For this review, take the finished solid that the model builds, in its own axes (mm). Coordinates: 2 decimals unless noted, no trailing zeros. Write each loop counter-clockwise with the first axis right and the second up, starting at its lowest first coordinate (ties: lowest second). Pieces come first, ordered by that corner, then holes. Notation, with made-up numbers: (49.5, 75.25) -> (81.5, 75.25) arc R7 ccw to (81.5, 82.25) -> close; hole circle Ø7 at (14, 58). An arc over 180 degrees is marked (long way). Put each result on its own line as item: value. Start each with the question number.
Item 1: Consider section C-C on x = 840. Give the boundary of the cut face in (y, z) (3 decimals), and give its area (3 significant figures).
Item 2: To check wall thickness, follow L1, parallel to X at y = 44.45, z = 6; L2, parallel to Y at x = 1365.25, z = 8; L3, parallel to X at y = 758.5, z = 14.75. State the ranges of each line that lie inside material, in increasing order.
Item 3: Consider section A-A on y = 698.5. Give the boundary of the cut face in (x, z) (3 decimals), and give its area (3 significant figures).
Item 4: Consider section B-B on z = 3.25. Give the boundary of the cut face in (x, y) (3 decimals).
Item 5: Insertion check: P1, Ø10, axis at x = 1365.25, y = 44.45, coming from the -Z side. The pin has a flat end and moves straight along its axis. Give the tip position at first contact, or say it passes through.
Autodesk Inventor part; units mm, degrees
ref_plane "YZ Plane" through (0, 0, 0) normal (1, 0, 0) x (0, 1, 0)
ref_plane "XZ Plane" through (0, 0, 0) normal (0, 1, 0) x (-1, 0, 0)
ref_plane "XY Plane" through (0, 0, 0) normal (0, 0, 1) x (1, 0, 0)
sketch "Sketch1" plane through (0, 0, 0) normal (0, 0, 1) x (1, 0, 0)
  line L0 (0, 0) -> (1428.75, 0)
  line L1 (1428.75, 1219.2) -> (0, 1219.2)
  line L2 (0, 1219.2) -> (0, 0)
  line L3 (0, 0) -> (1428.75, 0)
  line L4 (1428.75, 1219.2) -> (0, 1219.2)
  line L5 (0, 1219.2) -> (0, 0)
  line L6 (0, 1219.2) -> (1428.75, 1219.2)
  line L7 (1428.75, 1219.2) -> (1428.75, 0)
extrude "Extrusion1" add sketch "Sketch1" along normal blind 15.875
sketch "Sketch2" plane through (0, 0, 15.875) normal (0, 0, 1) x (1, 0, 0)
  circle A0 centre (714.375, 698.5) radius 152.4
extrude "Extrusion2" cut sketch "Sketch2" against normal blind 15.875
sketch "Sketch3" plane through (0, 0, 15.875) normal (0, 0, 1) x (1, 0, 0)
  line L0 (1428.75, 0) -> (1428.75, 1219.2)
  line L1 (0, 0) -> (63.5, 0)
  point P0 (1365.25, 44.45)
  point P1 (63.5, 44.45)
hole "Hole1" at (1365.25, 44.45, 15.875) at (63.5, 44.45, 15.875) direction (0, 0, -1) diameter 12.7 end through all
properties part number "56.25x48 Gyp"
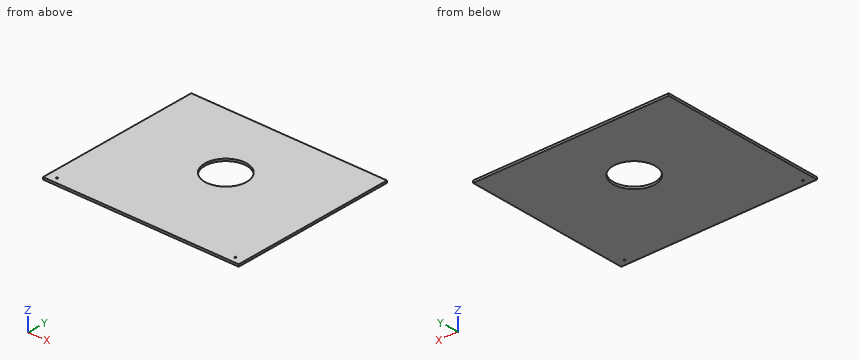
Return value:
1. outline: (0, 0) -> (612.221, 0) -> (612.221, 15.875) -> (0, 15.875) -> close; (784.779, 0) -> (1219.2, 0) -> (1219.2, 15.875) -> (784.779, 15.875) -> close
1. area: 16,600 mm^2
2. L1: 0 to 57.15, 69.85 to 1358.9, 1371.6 to 1428.75
2. L2: 0 to 38.1, 50.8 to 1219.2
2. L3: 0 to 574.28, 854.47 to 1428.75
3. outline: (0, 0) -> (561.975, 0) -> (561.975, 15.875) -> (0, 15.875) -> close; (866.775, 0) -> (1428.75, 0) -> (1428.75, 15.875) -> (866.775, 15.875) -> close
3. area: 17,800 mm^2
4. outline: (0, 0) -> (1428.75, 0) -> (1428.75, 1219.2) -> (0, 1219.2) -> close; hole circle Ø12.7 at (63.5, 44.45); hole circle Ø304.8 at (714.375, 698.5); hole circle Ø12.7 at (1365.25, 44.45)
5. P1: through
